Design review of the part built by this model. Coordinates are the model's own, in mm. A direction names the side the tool comes from. Coordinates: 2 decimals unless noted, no trailing zeros. Loops run counter-clockwise (first coordinate to the right, second up) from the corner with the lowest first, then second, coordinate; pieces in that order, holes last. Notation, with made-up numbers: (59, -11.75) - (70, -11.75) arc R15 cw to (70, -7.75) - close; hole circle Ø9 at (15.5, 45.5). An arc over 180 degrees is marked (long way). One line per question, with ' | ' between items.
from build123d import *

# Parameters (mm, degrees)
F1_DEPTH = 434
F2_W     = 50.4274696951
F2_H     = 227
F3_DEPTH = 132.001
F5_DEPTH = 25.4
F6_R     = 1


with BuildPart() as f1:
    # F0 (on Front) → F1 (new body)
    with BuildSketch(Plane.XZ):
        Polygon((-133.9674020287, 67), (-218.9674020287, 67), (-218.9674020287, 57), (-143.9674020287, 57), (-143.9674020287, -10), (191.0325979713, -10), (191.0325979713, -65), (201.0325979713, -65), (201.0325979713, 0), (-133.9674020287, 0), align=None)
    extrude(amount=F1_DEPTH)

    # F2 (on face) → F3 (cut, through all)
    with BuildSketch(Plane.XY.offset(67)):
        with Locations((-193.7536671811, -217)):
            Rectangle(F2_W, F2_H)
    extrude(amount=-F3_DEPTH, mode=Mode.SUBTRACT)

    # F4 (on face) → F5 (cut)
    with BuildSketch(Plane.YZ.offset(-133.9674020287)):
        with BuildLine():
            Line((-127.8944141269, 42), (-253.5, 42))
            ThreePointArc((-253.5, 42), (-259.5104076401, 39.5104076401), (-262, 33.5))
            ThreePointArc((-262, 33.5), (-259.5104076401, 27.4895923599), (-253.5, 25))
            Line((-253.5, 25), (-127.8944141269, 25))
            ThreePointArc((-127.8944141269, 25), (-121.8840064868, 27.4895923599), (-119.3944141269, 33.5))
            ThreePointArc((-119.3944141269, 33.5), (-121.8840064868, 39.5104076401), (-127.8944141269, 42))
        make_face()
    extrude(amount=-F5_DEPTH, mode=Mode.SUBTRACT)

    # F6
    f6_edges = [f1.edges().sort_by_distance(p)[0] for p in [
        (-193.753667, -103.5, 67),
        (-168.539932, -103.5, 62),
        (-168.539932, -217, 57),
        (-168.539932, -217, 67),
        (-218.967402, -51.75, 67),
        (-218.967402, -51.75, 57),
        (-218.967402, -103.5, 62),
        (-218.967402, 0, 62),
        (-176.467402, 0, 67),
        (-133.967402, -217, 67),
        (-218.967402, -382.25, 67),
        (-218.967402, -382.25, 57),
        (-218.967402, -330.5, 62),
        (-193.753667, -330.5, 57),
        (-193.753667, -330.5, 67),
        (-168.539932, -330.5, 62),
        (-176.467402, -434, 67),
        (-218.967402, -434, 62),
        (-181.467402, -434, 57),
        (-143.967402, -434, 23.5),
        (-133.967402, -434, 33.5),
        (-143.967402, -217, -10),
        (-143.967402, 0, 23.5),
        (-133.967402, 0, 33.5),
        (33.532598, 0, 0),
        (23.532598, 0, -10),
        (-181.467402, 0, 57),
        (33.532598, -434, 0),
        (23.532598, -434, -10),
        (-133.967402, -217, 0),
        (201.032598, -217, 0),
        (201.032598, -434, -32.5),
        (191.032598, -434, -37.5),
        (196.032598, -434, -65),
        (201.032598, -217, -65),
        (191.032598, -217, -65),
        (201.032598, 0, -32.5),
        (191.032598, 0, -37.5),
        (191.032598, -217, -10),
        (-193.753667, -103.5, 57),
    ]]
    fillet(f6_edges, radius=F6_R)


solid = f1.part
Q1. Take a section at D-D (z = -36). Give the boundary of the cut face in (x, y), plus the area to 3 significant figures.
Returned:
outline: (191.03, -433) arc R1 ccw to (192.03, -434) - (200.03, -434) arc R1 ccw to (201.03, -433) - (201.03, -1) arc R1 ccw to (200.03, 0) - (192.03, 0) arc R1 ccw to (191.03, -1) - close | area: 4,340 mm²
Q2. For pin 1 (4 mm diameter, centred on y = -231.5, z = 60.5, fed in from -X); pin 2 (5 mm diameter, centred on y = -387, z = 14, fed in from +X); pin 3 (20 mm diameter, centred on y = -136.5, z = 12.5, fed in from -X), all flat-tipped, find the tip position at first contact; note any pin that passes through.
Returned:
pin 1: stops at x = -168.54 | pin 2: stops at x = -133.97 | pin 3: stops at x = -143.97
Q3. Draft analysis for pull direction Z (two halves, no side actions). For faces 1 (the flat face through (36, -214, 0)), 2 (the flat face through (-10, 0, -4)), 3 (the flat face through (-139, -192, 25)), 4 (the flat face through (21, -214, -10)), state which applies: +Z half, -Z half, draft (parallel to the pull), parting line (faces both ways), or undercut.
Returned:
face 1: +Z half | face 2: draft | face 3: undercut | face 4: -Z half
Q4. Tool access review of faces 5 (the flat face through (-139, -190, 42)), 6 (the flat face through (-165, -214, 57)), 7 (the flat face through (-133.967, -214, 19)): name each direction out of +Z, -Z, +X, -X, +Y, -Y from which nothing blocks a thin tool from reaching the whole face with its end or side.
Returned:
face 5: +X, -X | face 6: -Z, -X, +Y, -Y | face 7: +Z, +X, +Y, -Y
Q5. To check wall thickness, follow line 1 along X through (y, z) = (-296.5, -31); line 2 along X through (y, z) = (-372, 30); line 3 along Z through (x, y) = (57, -31). State the ranges of each line that lie inside material, in increasing order.
Returned:
line 1: x = 191.03 to 201.03 | line 2: x = -143.97 to -133.97 | line 3: z = -10 to 0
Q6. Take a section at B-B (y = -304). Give the boundary of the cut face in (x, z).
Returned:
outline: (-168.54, 58) arc R1 ccw to (-167.54, 57) - (-143.97, 57) - (-143.97, -9) arc R1 ccw to (-142.97, -10) - (190.03, -10) arc R1 cw to (191.03, -11) - (191.03, -64) arc R1 ccw to (192.03, -65) - (200.03, -65) arc R1 ccw to (201.03, -64) - (201.03, -1) arc R1 ccw to (200.03, 0) - (-132.97, 0) arc R1 cw to (-133.97, 1) - (-133.97, 66) arc R1 ccw to (-134.97, 67) - (-167.54, 67) arc R1 ccw to (-168.54, 66) - close
Q7. Take a section at A-A (y = -178.5). Give the boundary of the cut face in (x, z).
Returned:
outline: (-168.54, 58) arc R1 ccw to (-167.54, 57) - (-143.97, 57) - (-143.97, 42) - (-133.97, 42) - (-133.97, 66) arc R1 ccw to (-134.97, 67) - (-167.54, 67) arc R1 ccw to (-168.54, 66) - close; (-143.97, -9) arc R1 ccw to (-142.97, -10) - (190.03, -10) arc R1 cw to (191.03, -11) - (191.03, -64) arc R1 ccw to (192.03, -65) - (200.03, -65) arc R1 ccw to (201.03, -64) - (201.03, -1) arc R1 ccw to (200.03, 0) - (-132.97, 0) arc R1 cw to (-133.97, 1) - (-133.97, 25) - (-143.97, 25) - close
Q8. Take a section at C-C (x = 143.5). Give the boundary of the cut face in (y, z).
Returned:
outline: (-434, -9) arc R1 ccw to (-433, -10) - (-1, -10) arc R1 ccw to (0, -9) - (0, -1) arc R1 ccw to (-1, 0) - (-433, 0) arc R1 ccw to (-434, -1) - close
